The listing builds one solid part. Answer for the finished solid, in the listing's coordinates (mm). A direction names the side the tool comes from. Round coordinates to 2 decimals unless told otherwise and drop trailing zeros. Order: outer loops, then holes, each group sorted by start corner. A loop starts at its lowest first (then second) coordinate and runs counter-clockwise, first axis right, second up. Notation, with made-up numbers: (42, 38) - (54, 38) arc R23 ccw to (54, 54) - close; hole circle Ø3 at (72.5, -29). An arc over 180 degrees is marked (long way). One line per item, written item: value. Start each with the question number.
1. Flat-ended cylindrical pins translate along their axes: P1, Ø4, axis at y = 27, z = -25.5, coming from the -X side; P2, Ø6, axis at x = -10, z = 23, coming from the -Y side; P3, Ø10, axis at x = -11, z = 2, coming from the +Y side; P4, Ø19, axis at y = 0, z = 0, coming from the +X side. Find the tip coordinate at first contact, or state that the pin passes through.
2. A tool of negligible diameter and unlimited length cuts with its end or side. For faces 4 (the flat face through (-14, 33, 11)), 5 (the cylindrical face through (0.28, -3.604, 11.446)), 6 (the flat face through (5, 22, 0)), from which of +Z, -Z, +X, -X, +Y, -Y can it reach the whole face along a straight path? Write none if from no direction.
3. Section A-A, the plane z = 0 is taken. Give the vertices of the cut face in (x, y).
4. For a pull along Z with two mould halves and no side action, classify faces 1 (the cylindrical face through (0.196, 22.818, -29.759)), 2 (the flat face through (-20, -10, -7)), 3 (the flat face through (-5, 22, 0)) as released by +Z, released by -Z, zero draft, split by the parting line, or undercut.
5. Section D-D, the plane x = -11.5 is taken. Give the vertices of the cut face in (y, z), then the cut area to 3 significant figures.
6. Straight lines are drawn through the part: line 1 (Y direction, x = 7, z = 0); line 2 (Y direction, x = 3.5, z = 0); line 3 (Y direction, x = -6, z = 0). For each, find the intervals that lie inside material, in ascending order.
7. Section C-C, the plane x = 15.5 is taken. Give the vertices of the cut face in (y, z).
from build123d import *

# Parameters (mm, degrees)
SKETCH1_W   = 40
SKETCH1_H   = 3
SKETCH1_W_2 = 10
SKETCH1_H_2 = 13
SKETCH1_W_3 = 28


with BuildPart() as part:
    # Sketch1 → Revolve1 (revolve)
    with BuildSketch(Plane.XY, mode=Mode.PRIVATE) as revolve1_sk:
        with Locations((0, -13.5)):
            Rectangle(SKETCH1_W, SKETCH1_H)
        Polygon((20, -15), (5, -20), (-5, -20), (-20, -15), align=None)
        with Locations((0, -26.5)):
            Rectangle(SKETCH1_W_2, SKETCH1_H_2)
        Polygon((5, -33), (14, -34.5), (-14, -34.5), (-5, -33), align=None)
        with Locations((0, -36)):
            Rectangle(SKETCH1_W_3, SKETCH1_H)
    revolve(revolve1_sk.sketch.rotate(Axis((0, 0, 0), (1, 0, 0)), 270), axis=Axis((0, 0, 0), (1, 0, 0)))


solid = part.part
Answer list:
1. P1: stops at x = -14
1. P2: stops at y = -31.72
1. P3: stops at y = 37.5
1. P4: passes through
2. face 4: -X
2. face 5: +X, -X
2. face 6: +X
3. outline: (-20, -15) - (-5, -20) - (-5, -33) - (-14, -34.5) - (-14, -37.5) - (14, -37.5) - (14, -34.5) - (5, -33) - (5, -20) - (20, -15) - (20, -12) - (-20, -12) - close; (-20, 12) - (20, 12) - (20, 15) - (5, 20) - (5, 33) - (14, 34.5) - (14, 37.5) - (-14, 37.5) - (-14, 34.5) - (-5, 33) - (-5, 20) - (-20, 15) - close
4. face 1: split by the parting line
4. face 2: zero draft
4. face 3: undercut
5. outline: circle Ø75 at (0, 0); circle Ø35.67 at (0, 0); hole circle Ø68.17 at (0, 0); hole circle Ø24 at (0, 0)
5. area: 1,320 mm²
6. line 1: y = -37.5 to -33.33, -19.33 to -12, 12 to 19.33, 33.33 to 37.5
6. line 2: y = -37.5 to -12, 12 to 37.5
6. line 3: y = -37.5 to -33.17, -19.67 to -12, 12 to 19.67, 33.17 to 37.5
7. outline: circle Ø33 at (0, 0); hole circle Ø24 at (0, 0)
